Check sheet for the drawn part. Datum: minimum x, y, z corner. Units: mm. Round coordinates to 2 decimals unless told otherwise and drop trailing zeros. Write each loop counter-clockwise with the first axis right and the second up, starting at its lowest first coordinate (ties: lowest second). Pieces come first, ordered by that corner, then holes. Notation, with made-up numbers: (21, 86) -> (30, 86) arc R10 ccw to (30, 95) -> close; hole circle Ø2 at (-19, -21). An arc over 180 degrees is marked (long way). One line per item, written item: value. Start each with the question number.
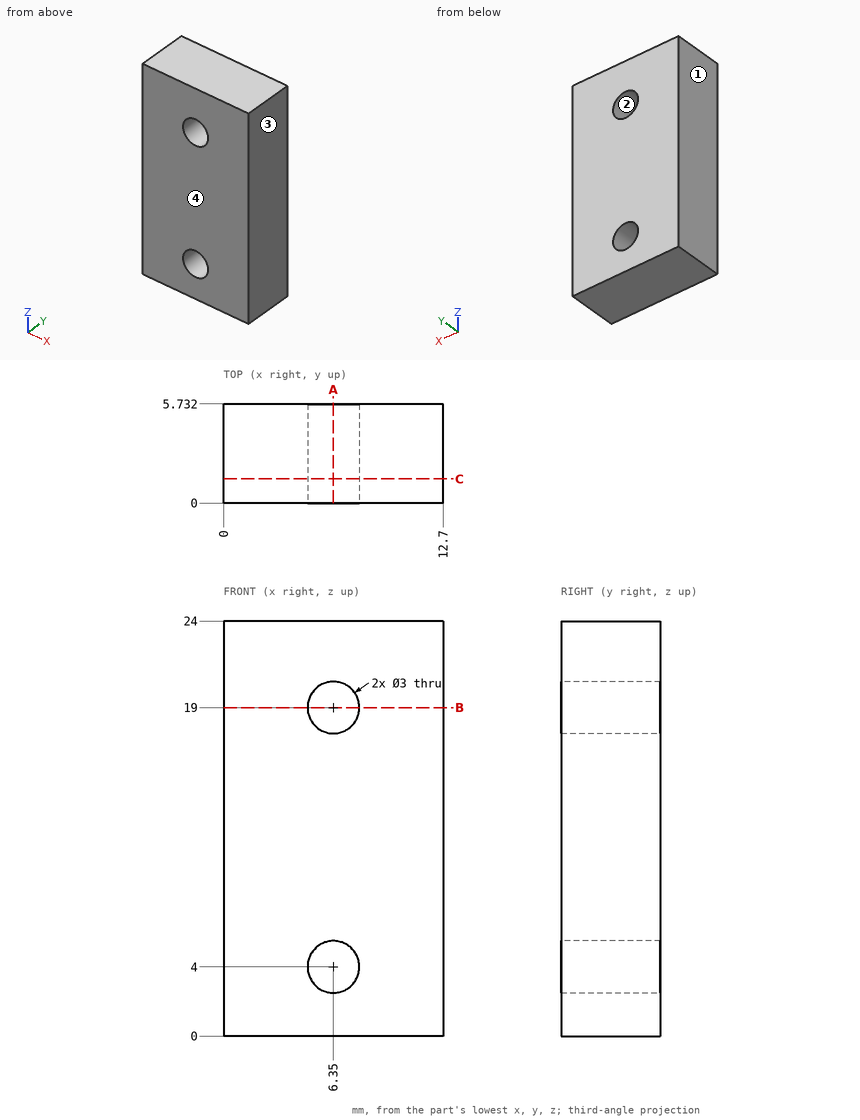
1. Depth check by flat-ended pin: pin 1 Ø3.5 at (x, z) = (6.35, 4) entering from +Y; pin 2 Ø2.5 at (x, z) = (6.35, 19) entering from +Y (3 decimals). Enter the tip coordinate at first touch or a pass-through.
2. Cross-section at B-B (z = 19). Record the cut outline in (x, y), plus the area to 3 significant figures.
3. Cross-section at C-C (y = 1.4). Record the cut outline in (x, z).
4. Material ranges on probe 1 along X at (y, z) = (4.05, 4); probe 2 along Z at (x, y) = (6, 3.4); probe 3 along X at (y, z) = (2.6, 17.75), recorded low to high.
5. Cross-section at A-A (x = 6.35). Record the cut outline in (y, z).
6. Release check for a two-part mould opening along X. For the marked faces 1, 2, 3 and 4 record: +X half, -X half, draft (parallel to the pull), parting line (faces both ways), or undercut.
Working result:
1. pin 1: stops at y = 5.73
1. pin 2: passes through
2. outline: (0, 0) -> (4.85, 0) -> (4.85, 5.73) -> (0, 5.73) -> close; (7.85, 0) -> (12.7, 0) -> (12.7, 5.73) -> (7.85, 5.73) -> close
2. area: 55.6 mm^2
3. outline: (0, 0) -> (12.7, 0) -> (12.7, 24) -> (0, 24) -> close; hole circle Ø3 at (6.35, 4); hole circle Ø3 at (6.35, 19)
4. probe 1: x = 0 to 4.85, 7.85 to 12.7
4. probe 2: z = 0 to 2.54, 5.46 to 17.54, 20.46 to 24
4. probe 3: x = 0 to 5.52, 7.18 to 12.7
5. outline: (0, 0) -> (5.73, 0) -> (5.73, 2.5) -> (0, 2.5) -> close; (0, 5.5) -> (5.73, 5.5) -> (5.73, 17.5) -> (0, 17.5) -> close; (0, 20.5) -> (5.73, 20.5) -> (5.73, 24) -> (0, 24) -> close
6. face 1: -X half
6. face 2: undercut
6. face 3: +X half
6. face 4: draft
